```python
from build123d import *

# Parameters (mm, degrees)
F0_W       = 80.01
F0_H       = 32.992
F1_DEPTH   = 48.175
F3_DEPTH   = 32.992
F4_R       = 12.5
F5_DEPTH   = 34.036
F6_R       = 3
F7_DEPTH   = 7.874
F8_W       = 80.01
F8_H       = 96.35
F8_R       = 3
F8_R_2     = 12.5
F9_DEPTH   = 15
F12_DEPTH  = 5.005
F14_DEPTH  = 4.454
F16_DEPTH  = 5.005
F17_R      = 27
F19_R      = 52.451
F21_DEPTH  = 21
F21_FACE_R = 52.451
F23_R      = 44.45
F27_W      = 67
F27_H      = 67
F28_DEPTH  = 80.772
F29_W      = 94
F29_H      = 94
F30_DEPTH  = 45
F31_SIZE   = 7.62
F32_SIZE   = 2.54
F33_SIZE   = 5.08


with BuildPart() as f1:
    # F0 (on Top) → F1 (new body, symmetric)
    with BuildSketch(Plane.XY):
        Rectangle(F0_W, F0_H)
    extrude(amount=F1_DEPTH, both=True)

    # F2 (on face) → F3 (cut, through all)
    with BuildSketch(Plane.XZ.offset(16.496)):
        with BuildLine():
            Line((-2.5, 0.579), (-2.5, -2.1826515847))
            ThreePointArc((-2.5, -2.1826515847), (0, -15.721), (2.5, -2.1826515847))
            Line((2.5, -2.1826515847), (2.5, 0.579))
            Line((2.5, 0.579), (-2.5, 0.579))
        make_face()
    extrude(amount=-F3_DEPTH, mode=Mode.SUBTRACT)

    # F4 (on Front) → F5 (join, symmetric)
    with BuildSketch(Plane.XZ):
        with Locations((0, -8.721)):
            Circle(F4_R)
        with BuildLine():
            ThreePointArc((2.5, -2.1826515847), (0, -15.721), (-2.5, -2.1826515847))
            Line((-2.5, -2.1826515847), (-2.5, 0.579))
            Line((-2.5, 0.579), (2.5, 0.579))
            Line((2.5, 0.579), (2.5, -2.1826515847))
        make_face(mode=Mode.SUBTRACT)
    extrude(amount=F5_DEPTH, both=True)

    # F6 (on face) → F7 (cut)
    with BuildSketch(Plane.XZ.offset(16.496)):
        with Locations((0, 21.251)):
            Circle(F6_R)
        with Locations((-29.972, -8.721)):
            Circle(F6_R)
        with Locations((0, -38.693)):
            Circle(F6_R)
        with Locations((29.972, -8.721)):
            Circle(F6_R)
    extrude(amount=-F7_DEPTH, mode=Mode.SUBTRACT)

    # F10: F9 across plane


with BuildPart() as f9:
    # F8 (on face) → F9 (new body)
    with BuildSketch(Plane.XZ.offset(16.496)):
        Rectangle(F8_W, F8_H)
        Polygon((-1.5, 43.17), (-1.5, 26.279), (1.5, 26.279), (1.5, 43.17), (35, 43.17), (35, -2.721), (35, -14.721), (35, -43.721), (6, -43.721), (-6, -43.721), (-35, -43.721), (-35, -14.721), (-35, -2.721), (-35, 43.17), align=None, mode=Mode.SUBTRACT)
        with BuildLine():
            Line((-6, 26.279), (-6, 18.1164738006))
            ThreePointArc((-6, 18.1164738006), (-19.4454364826, 10.7244364826), (-26.8374738006, -2.721))
            Line((-26.8374738006, -2.721), (-35, -2.721))
            Line((-35, -2.721), (-35, -14.721))
            Line((-35, -14.721), (-26.8374738006, -14.721))
            ThreePointArc((-26.8374738006, -14.721), (-19.4454364826, -28.1664364826), (-6, -35.5584738006))
            Line((-6, -35.5584738006), (-6, -43.721))
            Line((-6, -43.721), (6, -43.721))
            Line((6, -43.721), (6, -35.5584738006))
            ThreePointArc((6, -35.5584738006), (19.4454364826, -28.1664364826), (26.8374738006, -14.721))
            Line((26.8374738006, -14.721), (35, -14.721))
            Line((35, -14.721), (35, -2.721))
            Line((35, -2.721), (26.8374738006, -2.721))
            ThreePointArc((26.8374738006, -2.721), (19.4454364826, 10.7244364826), (6, 18.1164738006))
            Line((6, 18.1164738006), (6, 26.279))
            Line((6, 26.279), (1.5, 26.279))
            Line((1.5, 26.279), (-1.5, 26.279))
            Line((-1.5, 26.279), (-6, 26.279))
        make_face()
        with Locations((-29.972, -8.721)):
            Circle(F8_R, mode=Mode.SUBTRACT)
        with Locations((0, -38.693)):
            Circle(F8_R, mode=Mode.SUBTRACT)
        with Locations((0, -8.721)):
            Circle(F8_R_2, mode=Mode.SUBTRACT)
        with Locations((29.972, -8.721)):
            Circle(F8_R, mode=Mode.SUBTRACT)
        with Locations((0, 21.251)):
            Circle(F8_R, mode=Mode.SUBTRACT)
    extrude(amount=F9_DEPTH)


with BuildPart() as f1_1:
    add(f1.part)
    add(f9.part.mirror(Plane.XZ))


with BuildPart() as f12_tool:
    # F11 (on face) → F12 (new body, through all)
    with BuildSketch(Plane.XY.offset(48.175)):
        with BuildLine():
            Line((-30.607, -21.971), (-30.607, -31.496))
            Line((-30.607, -31.496), (-23.495, -31.496))
            Line((-23.495, -31.496), (-23.495, -21.971))
            ThreePointArc((-23.495, -21.971), (-27.051, -18.415), (-30.607, -21.971))
        make_face()
        with BuildLine():
            Line((30.607, -31.496), (30.607, -21.971))
            ThreePointArc((30.607, -21.971), (27.051, -18.415), (23.495, -21.971))
            Line((23.495, -21.971), (23.495, -31.496))
            Line((23.495, -31.496), (30.607, -31.496))
        make_face()
        with BuildLine():
            Line((-30.607, 31.496), (-30.607, 21.971))
            ThreePointArc((-30.607, 21.971), (-27.051, 18.415), (-23.495, 21.971))
            Line((-23.495, 21.971), (-23.495, 31.496))
            Line((-23.495, 31.496), (-30.607, 31.496))
        make_face()
        with BuildLine():
            Line((30.607, 21.971), (30.607, 31.496))
            Line((30.607, 31.496), (23.495, 31.496))
            Line((23.495, 31.496), (23.495, 21.971))
            ThreePointArc((23.495, 21.971), (27.051, 18.415), (30.607, 21.971))
        make_face()
    extrude(amount=-F12_DEPTH)


with BuildPart() as f1_2:
    add(f1_1.part)

    # F12: cut by f12_tool
    add(f12_tool.part, mode=Mode.SUBTRACT)


with BuildPart() as f9_1:
    add(f9.part)

    # F12: cut by f12_tool
    add(f12_tool.part, mode=Mode.SUBTRACT)


with BuildPart() as f14_tool:
    # F13 (on face) → F14 (new body, through all)
    with BuildSketch(Plane(origin=(0, 0, -48.175), x_dir=(1, 0, 0), z_dir=(0, 0, -1))):
        with BuildLine():
            ThreePointArc((-30.607, 21.971), (-27.051, 18.415), (-23.495, 21.971))
            Line((-23.495, 21.971), (-23.495, 31.496))
            Line((-23.495, 31.496), (-30.607, 31.496))
            Line((-30.607, 31.496), (-30.607, 21.971))
        make_face()
        with BuildLine():
            Line((23.495, 31.496), (23.495, 21.971))
            ThreePointArc((23.495, 21.971), (27.051, 18.415), (30.607, 21.971))
            Line((30.607, 21.971), (30.607, 31.496))
            Line((30.607, 31.496), (23.495, 31.496))
        make_face()
        with BuildLine():
            ThreePointArc((30.607, -21.971), (27.051, -18.415), (23.495, -21.971))
            Line((23.495, -21.971), (23.495, -31.496))
            Line((23.495, -31.496), (30.607, -31.496))
            Line((30.607, -31.496), (30.607, -21.971))
        make_face()
        with BuildLine():
            Line((-30.607, -21.971), (-30.607, -31.496))
            Line((-30.607, -31.496), (-23.495, -31.496))
            Line((-23.495, -31.496), (-23.495, -21.971))
            ThreePointArc((-23.495, -21.971), (-27.051, -18.415), (-30.607, -21.971))
        make_face()
    extrude(amount=-F14_DEPTH)


with BuildPart() as f1_3:
    add(f1_2.part)

    # F14: cut by f14_tool
    add(f14_tool.part, mode=Mode.SUBTRACT)


with BuildPart() as f9_2:
    add(f9_1.part)

    # F14: cut by f14_tool
    add(f14_tool.part, mode=Mode.SUBTRACT)


with BuildPart() as f16_tool:
    # F15 (on face) → F16 (new body, through all)
    with BuildSketch(Plane(origin=(-40.005, 0, 0), x_dir=(0, -1, 0), z_dir=(-1, 0, 0))):
        with BuildLine():
            Line((31.496, 32.004), (31.496, 39.116))
            Line((31.496, 39.116), (21.971, 39.116))
            ThreePointArc((21.971, 39.116), (18.415, 35.56), (21.971, 32.004))
            Line((21.971, 32.004), (31.496, 32.004))
        make_face()
        with BuildLine():
            ThreePointArc((-21.971, 32.004), (-18.415, 35.56), (-21.971, 39.116))
            Line((-21.971, 39.116), (-31.496, 39.116))
            Line((-31.496, 39.116), (-31.496, 32.004))
            Line((-31.496, 32.004), (-21.971, 32.004))
        make_face()
        with BuildLine():
            Line((-31.496, -32.004), (-31.496, -39.116))
            Line((-31.496, -39.116), (-21.971, -39.116))
            ThreePointArc((-21.971, -39.116), (-18.415, -35.56), (-21.971, -32.004))
            Line((-21.971, -32.004), (-31.496, -32.004))
        make_face()
        with BuildLine():
            ThreePointArc((21.971, -32.004), (18.415, -35.56), (21.971, -39.116))
            Line((21.971, -39.116), (31.496, -39.116))
            Line((31.496, -39.116), (31.496, -32.004))
            Line((31.496, -32.004), (21.971, -32.004))
        make_face()
    extrude(amount=-F16_DEPTH)


with BuildPart() as f1_4:
    add(f1_3.part)

    # F16: cut by f16_tool
    add(f16_tool.part, mode=Mode.SUBTRACT)



with BuildPart() as f9_3:
    add(f9_2.part)

    # F16: cut by f16_tool
    add(f16_tool.part, mode=Mode.SUBTRACT)


with BuildPart() as f1_5:
    add(f1_4.part)

    add(f9_3.part)  # F20 merges F9
    # F17 (on face) → F20 section 0
    with BuildSketch(Plane.YZ.offset(40.005)):
        with Locations((0, 22.267)):
            Circle(F17_R)
    # F19 (on offset) → F20 section 1
    with BuildSketch(Plane(origin=(48.995, 0, 0), x_dir=(0, -1, 0), z_dir=(-1, 0, 0))):
        with Locations((0, 22.267)):
            Circle(F19_R)
    loft()

    # F19 (on offset) → F21 (join)
    with BuildSketch(Plane(origin=(48.995, 0, 0), x_dir=(0, -1, 0), z_dir=(-1, 0, 0))):
        with Locations((0, 22.267)):
            Circle(F19_R)
    extrude(amount=-F21_DEPTH)

    # F21_face (on face) → F24 section 0
    with BuildSketch(Plane(origin=(69.995, 0, 22.267), x_dir=(0, -1, 0), z_dir=(1, 0, 0))):
        Circle(F21_FACE_R)
    # F23 (on offset) → F24 section 1
    with BuildSketch(Plane.YZ.offset(77.995)):
        with Locations((0, 22.267)):
            Circle(F23_R)
    loft()

    # F25 (on Front) → F26 (revolve)
    with BuildSketch(Plane.XZ):
        Polygon((84.9672986563, 66.717), (77.995, 66.717), (77.995, 22.267), (301.995, 22.267), (301.995, 75.0546455383), (289.995, 79.6519890428), (254.995, 79.6519890428), (251.252396116, 82.4864879847), (233.252396116, 82.4864879847), (233.252396116, 71.4864879847), (104.9230620265, 71.4864879847), (90.6504243612, 69.2906975746), align=None)
    revolve(axis=Axis((189.995, 0, 22.267), (-1, 0, 0)))

    # F27 (on Top) → F28 (join)
    with BuildSketch(Plane.XY):
        with Locations((170.495, 0)):
            Rectangle(F27_W, F27_H)
    extrude(amount=F28_DEPTH)

    # F29 (on face) → F30 (join)
    with BuildSketch(Plane.XY.offset(80.772)):
        with Locations((170.495, 0)):
            Rectangle(F29_W, F29_H)
    extrude(amount=F30_DEPTH)

    # F31
    f31_edges = [f1_5.edges().sort_by_distance(p)[0] for p in [
        (170.495, 47, 125.772),
        (123.495, 0, 125.772),
        (170.495, -47, 125.772),
        (217.495, 0, 125.772),
    ]]
    chamfer(f31_edges, length=F31_SIZE)

    # F32
    f32_edges = [f1_5.edges().sort_by_distance(p)[0] for p in [
        (170.495, 47, 80.772),
        (217.495, 0, 80.772),
        (123.495, 0, 80.772),
        (170.495, -47, 80.772),
        (203.995, 0, 80.772),
        (170.495, 33.5, 80.772),
        (136.995, 0, 80.772),
        (170.495, -33.5, 80.772),
    ]]
    chamfer(f32_edges, length=F32_SIZE)

    # F33
    f33_edges = [f1_5.edges().sort_by_distance(p)[0] for p in [
        (-40.005, 0, 48.175),
        (-40.005, 0, -48.175),
        (40.005, 0, -48.175),
    ]]
    chamfer(f33_edges, length=F33_SIZE)


solid = f1_5.part
```
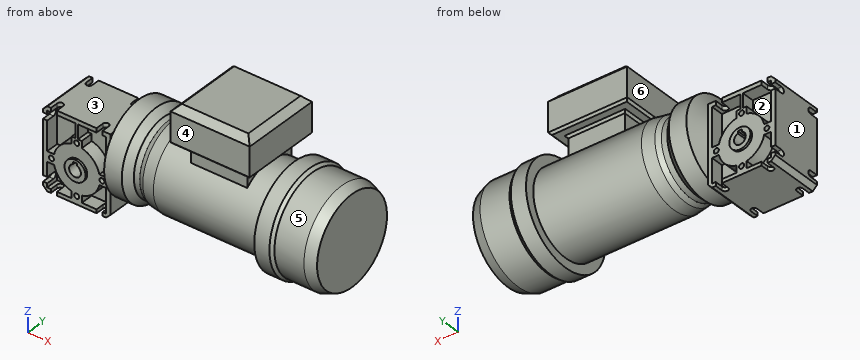
Build history of the part. All positions in model axes, mm. Face numbers are marked on the shaded views. A direction names the side the tool comes from. Coordinates: 2 decimals unless noted, no trailing zeros. Order: outer loops, then holes, each group sorted by start corner. A loop starts at its lowest first (then second) coordinate and runs counter-clockwise, first axis right, second up.
Item 1: Drill centre lines: L1, parallel to X at y = 29.5, z = 21 (3 decimals); L2, parallel to X at y = 20, z = -29 (1 decimal); L3, parallel to X at y = 28.5, z = 45 (3 decimals). Where is each one in solid material? Low to high.
Filled in:
L1: x = -40.005 to -35, -6 to -2.989, 2.989 to 6, 35 to 40.005, 40.898 to 301.995
L2: x = -40 to -35, -18.6 to 18.6, 35 to 40, 233.3 to 296.1
L3: x = -38.1 to -30.607, -23.495 to 23.495, 30.607 to 40.005, 43.345 to 301.995
Item 2: Tool access for the marked faces 4, 5 and 6: list every direction of +Z, -Z, +X, -X, +Y, -Y with a clear straight run to the whole face (end or side of a thin tool).
Filled in:
face 4: +Z, +X, -X, -Y
face 5: +X
face 6: +Z, -X, +Y, -Y
Item 3: Drop flat-ended pins along their axis: pin 1 Ø5 at (y, z) = (24.5, 70) entering from -X; pin 2 Ø1.3 at (x, y) = (-3.5, -27.5) entering from +Z (3 decimals); pin 3 Ø5 at (x, z) = (0, -38.693) entering from -Y. Give the stop position or say it passes through.
Filled in:
pin 1: stops at x = 48.54
pin 2: stops at z = 48.175
pin 3: stops at y = -8.62
Item 4: Saw through at A-A on x = 228.5. List the corners of the cut face in (y, z).
Filled in:
outline: circle Ø98.44 at (0, 22.27)
Item 5: Mould opens along X. For the marked faces 1, 2 and 3 say: released by +X, released by -X, zero draft, split by the parting line, or undercut.
Filled in:
face 1: released by -X
face 2: undercut
face 3: zero draft
